Verification items for the finished model (mm, model axes). A direction names the side the tool comes from. Give positions to 0.01 mm unless a question says otherwise; leave off trailing zeros. Loops run counter-clockwise (first coordinate to the right, second up) from the corner with the lowest first, then second, coordinate; pieces in that order, holes last. Notation, with made-up numbers: (89, 30.5) - (134, 30.5) arc R16 ccw to (134, 37.5) - close; hole circle Ø6 at (67, 81). An arc over 180 degrees is marked (long way). One line per question, with ' | ' between items. Start each with the question number.
1. Depth check by flat-ended pin: pin 1 Ø4 at (x, y) = (-2, 11) entering from -Z; pin 2 Ø3.5 at (x, z) = (-10.5, 11) entering from -Y; pin 3 Ø6 at (x, y) = (-8, -2) entering from +Z; pin 4 Ø5.5 at (x, z) = (-11, 11.5) entering from +Y. Enter the tip coordinate at first touch or a pass-through.
2. Thickness scan on line 1 along Y through (x, z) = (-14.5, 1.25); line 2 along Y through (x, z) = (2, 7); line 3 along Y through (x, z) = (-2.5, 6). Record the ranges inside material, lowest first. Write a range as from..to.
3. Section check D-D, the plane y = 0. Enter the section's corners in (x, z), then the cut area to 3 significant figures.
4. Section check C-C, the plane z = 18.25. Enter the section's corners in (x, y), then the cut area to 3 significant figures.
5. Section check A-A, the plane y = 12.5. Enter the section's corners in (x, z) (3 decimals).
6. Mould release check, pull along Y, two halves, no side actions. Record for faces 1 (the face through (-9, 13.5, 10)), 2 (the face through (-17.5, 0, 1)), 3 (the face through (6, -10.25, 13)), 4 (the face through (-14, 14, 1.5)): +Y half, -Y half, draft (parallel to the pull), parting line (faces both ways), or undercut.
7. Section check B-B, the plane x = -10.5. Enter the section's corners in (y, z) (3 decimals), then the cut area to 3 significant figures.
8. Tool access check on faces 5 (the face through (6, 8, 5)), 6 (the face through (-12.517, 12.24, 0.74)), 7 (the face through (-7.7, -14.2, 13.1)). Record the directions out of +Z, -Z, +X, -X, +Y, -Y that give a thin tool (end or side, any length) a straight path to the whole face; none if there is none.
from build123d import *

# Parameters (mm, degrees)
SKETCH1_W              = 35
SKETCH1_H              = 20
BASE_PLATE_DEPTH       = 3
SKETCH2_W              = 35
SKETCH2_H              = 5
SIDE_WALLS_DEPTH       = 23
SKETCH4_R              = 1.1
SKETCH4_R_2            = 1.25
M2_SCREWS_DEPTH        = 23
SKETCH6_W              = 5
SKETCH6_H              = 20
RETURN_STOPPER_DEPTH   = 4.5
SKETCH9_W              = 12
SKETCH9_H              = 16
BOSS_EXTRUDE1_DEPTH    = 4.5
SKETCH7_R              = 7.75
MAGNET_POCKET_DEPTH    = 6
SKETCH8_R              = 2
M2_SCREW_HEAD_DEPTH    = 1.5
M3_ACHSLE_DEPTH        = 39.213217609
M3_ACHSLE_DEPTH_BACK   = 39.213217609
SKETCH5_R              = 1.625
SKETCH14_R             = 3.5
CUT_EXTRUDE1_DEPTH     = 1.5
CUT_EXTRUDE2_START     = -1.5
SKETCH15_R             = 3.5
CUT_EXTRUDE2_DEPTH     = 1.5
FILLET1_R              = 1.5
LEAVER_START           = -0.25
SKETCH11_W             = 22
SKETCH11_H             = 15.5
LEAVER_SPACE_DEPTH     = 20.5
SKETCH12_W             = 17
SKETCH12_H             = 4.5
MORE_SPACE_LEFT_DEPTH  = 0.25
SKETCH13_W             = 17
SKETCH13_H             = 4.5
MORE_SPACE_RIGHT_DEPTH = 0.25
FILLET2_R              = 0.75
FILLET3_R              = 0.75
FILLET4_R              = 0.75
FILLET5_R              = 0.5
CHAMFER1_SIZE          = 13.050517742
CHAMFER1_SIZE_2        = 4.75


with BuildPart() as part:
    # Sketch1 → Base Plate (new body)
    with BuildSketch(Plane.XY):
        Rectangle(SKETCH1_W, SKETCH1_H)
    extrude(amount=BASE_PLATE_DEPTH)

    # Sketch2 → Side Walls (add)
    with BuildSketch(Plane(origin=(0, 0, 0), x_dir=(1, 0, 0), z_dir=(0, 0, -1))):
        with Locations((0, -12.5)):
            Rectangle(SKETCH2_W, SKETCH2_H)
        with Locations((0, 12.5)):
            Rectangle(SKETCH2_W, SKETCH2_H)
    extrude(amount=-SIDE_WALLS_DEPTH)

    # Sketch4 → M2 Screws (cut)
    with BuildSketch(Plane.XY.offset(23)):
        with Locations((-14.5, -12.5)):
            Circle(SKETCH4_R)
        with Locations((7.5, -12.5)):
            Circle(SKETCH4_R)
        with Locations((7.5, 12.5)):
            Circle(SKETCH4_R_2)
        with Locations((-14.5, 12.5)):
            Circle(SKETCH4_R_2)
    extrude(amount=-M2_SCREWS_DEPTH, mode=Mode.SUBTRACT)

    # Sketch6 → Return Stopper (add)
    with BuildSketch(Plane.XY.offset(3)):
        with Locations((15, 0)):
            Rectangle(SKETCH6_W, SKETCH6_H)
    extrude(amount=RETURN_STOPPER_DEPTH)

    # Sketch9 → Boss-Extrude1 (add)
    with BuildSketch(Plane.XY.offset(3)):
        with Locations((6.5, 0)):
            Rectangle(SKETCH9_W, SKETCH9_H)
    extrude(amount=BOSS_EXTRUDE1_DEPTH)

    # Sketch7 → Magnet Pocket (cut)
    with BuildSketch(Plane(origin=(0, 0, 0), x_dir=(-1, 0, 0), z_dir=(0, 0, 1))):
        with Locations(Location((-8.75, 0, 0), (0, 0, 90))):
            Circle(SKETCH7_R)
    extrude(amount=MAGNET_POCKET_DEPTH, mode=Mode.SUBTRACT)

    # Sketch8 → M2 Screw Head (cut)
    with BuildSketch(Plane(origin=(0, 0, 0), x_dir=(1, 0, 0), z_dir=(0, 0, -1))):
        with Locations(Location((7.5, -12.5, 0), (0, 0, 270))):
            Circle(SKETCH8_R)
        with Locations(Location((-14.5, -12.5, 0), (0, 0, 270))):
            Circle(SKETCH8_R)
        with Locations(Location((7.5, 12.5, 0), (0, 0, 270))):
            Circle(SKETCH8_R)
        with Locations(Location((-14.5, 12.5, 0), (0, 0, 270))):
            Circle(SKETCH8_R)
    extrude(amount=-M2_SCREW_HEAD_DEPTH, mode=Mode.SUBTRACT)

    # Sketch5 → M3 Achsle (cut, two sides: drawn at the far end of the back side and taken through both)
    with BuildSketch(Plane.XZ.offset(-10).offset(-M3_ACHSLE_DEPTH_BACK)):
        with Locations((-10.5, 11)):
            Circle(SKETCH5_R)
    extrude(amount=M3_ACHSLE_DEPTH + M3_ACHSLE_DEPTH_BACK, mode=Mode.SUBTRACT)

    # Sketch14 → Cut-Extrude1 (cut)
    with BuildSketch(Plane(origin=(0, 15, 0), x_dir=(-1, 0, 0), z_dir=(0, 1, 0))):
        with Locations((10.5, 11)):
            Circle(SKETCH14_R)
    extrude(amount=-CUT_EXTRUDE1_DEPTH, mode=Mode.SUBTRACT)

    # Sketch15 → Cut-Extrude2 (cut)
    with BuildSketch(Plane.XZ.offset(15).offset(CUT_EXTRUDE2_START)):
        with Locations(Location((-10.5, 11, 0), (0, 0, 180))):
            Circle(SKETCH15_R)
    extrude(amount=CUT_EXTRUDE2_DEPTH, mode=Mode.SUBTRACT)

    # Fillet1
    fillet1_edges = [part.edges().sort_by_distance(p)[0] for p in [
        (0.5, 0, 7.5),
    ]]
    fillet(fillet1_edges, radius=FILLET1_R)

    # Sketch11 → Leaver Space (cut)
    with BuildSketch(Plane.XZ.offset(-10).offset(LEAVER_START)):
        with Locations((6.5, 15.25)):
            Rectangle(SKETCH11_W, SKETCH11_H)
    extrude(amount=LEAVER_SPACE_DEPTH, mode=Mode.SUBTRACT)

    # Sketch12 → More Space left (cut)
    with BuildSketch(Plane.XZ.offset(-10)):
        with Locations((4, 5.25)):
            Rectangle(SKETCH12_W, SKETCH12_H)
    extrude(amount=-MORE_SPACE_LEFT_DEPTH, mode=Mode.SUBTRACT)

    # Sketch13 → More Space right (cut)
    with BuildSketch(Plane(origin=(0, -10, 0), x_dir=(-1, 0, 0), z_dir=(0, 1, 0))):
        with Locations((-4, 5.25)):
            Rectangle(SKETCH13_W, SKETCH13_H)
    extrude(amount=-MORE_SPACE_RIGHT_DEPTH, mode=Mode.SUBTRACT)

    # Fillet2
    # the kernel refuses this fillet: 0.75 mm, written as the material it takes off along each edge
    with BuildSketch(Plane(origin=(19.375, 15, 0), x_dir=(0, -1, 0), z_dir=(-1, 0, 0))) as fillet2_piece_1:
        with BuildLine():
            CenterArc((FILLET2_R, FILLET2_R), FILLET2_R, 180, 90)
            Line((0, FILLET2_R), (0, 0))
            Line((0, 0), (FILLET2_R, 0))
        make_face()
    extrude(amount=38.75, mode=Mode.SUBTRACT)

    # Fillet3
    # the kernel refuses this fillet: 0.75 mm, written as the material it takes off along each edge
    with BuildSketch(Plane(origin=(-19.375, -15, 0), x_dir=(0, 1, 0), z_dir=(1, 0, 0))) as fillet3_piece_1:
        with BuildLine():
            CenterArc((FILLET3_R, FILLET3_R), FILLET3_R, 180, 90)
            Line((0, FILLET3_R), (0, 0))
            Line((0, 0), (FILLET3_R, 0))
        make_face()
    extrude(amount=38.75, mode=Mode.SUBTRACT)

    # Fillet4
    fillet4_edges = [part.edges().sort_by_distance(p)[0] for p in [
        (-17.5, -15, 11.875),
        (-17.5, 0, 0),
        (-17.5, 14.780330086, 0.219669914),
        (-17.5, -14.780330086, 0.219669914),
        (-17.5, 15, 11.875),
    ]]
    fillet(fillet4_edges, radius=FILLET4_R)

    # Fillet5
    fillet5_edges = [part.edges().sort_by_distance(p)[0] for p in [
        (17.5, -15, 11.875),
        (17.5, 14.780330086, 0.219669914),
        (17.5, 0, 0),
        (17.5, -14.780330086, 0.219669914),
        (17.5, 15, 11.875),
    ]]
    fillet(fillet5_edges, radius=FILLET5_R)

    # Chamfer1
    # the kernel refuses this chamfer: 13.050517742, 4.75 mm, written as the material it takes off along each edge
    with BuildSketch(Plane(origin=(17.5, -48.355584384, 23), x_dir=(0.013184058198645798, 0, -0.9999130865277316), z_dir=(0, 1, 0))) as chamfer1_piece_1:
        Polygon((CHAMFER1_SIZE * 0.999913086559, CHAMFER1_SIZE * 0.0131840581991), (-CHAMFER1_SIZE_2 * 0.0131840581986, CHAMFER1_SIZE_2 * 0.999913086528), (0, 0), align=None)
    extrude(amount=71.961168769, mode=Mode.SUBTRACT)
    with BuildSketch(Plane(origin=(17.5, -23.605584384, 23), x_dir=(-0.9950833631817486, 0, 0.09904090225205059), z_dir=(0, 1, 0))) as chamfer1_piece_2:
        Polygon((CHAMFER1_SIZE_2 * 0.995083363182, -CHAMFER1_SIZE_2 * 0.0990409022521), (-CHAMFER1_SIZE * 0.0990409022552, -CHAMFER1_SIZE * 0.995083363213), (0, 0), align=None)
    extrude(amount=71.961168769, mode=Mode.SUBTRACT)


solid = part.part
Results list:
1) pin 1: z = 0 | pin 2: y = -13.5 | pin 3: z = 3 | pin 4: y = 13.5
2) line 1: -15..-14.5, -10.5..10.5, 14.5..15 | line 2: -15..-10.25, -8..8, 10.25..15 | line 3: -15..-10.25, 10.25..15
3) outline: (-17.5, 0.75) arc R0.75 ccw to (-16.75, 0) - (1, 0) - (1, 6) - (16.5, 6) - (16.5, 0) - (17, 0) arc R0.5 ccw to (17.5, 0.5) - (17.5, 7.5) - (2, 7.5) arc R1.5 ccw to (0.5, 6) - (0.5, 3) - (-17.5, 3) - close | area: 87.8 mm²
4) outline: (-17.5, -14.25) arc R0.75 ccw to (-16.75, -15) - (14.48, -15) - (14.48, -10.25) - (-4.5, -10.25) - (-4.5, -10) - (-17.5, -10) - close; (-17.5, 10) - (-4.5, 10) - (-4.5, 10.25) - (14.48, 10.25) - (14.48, 15) - (-16.75, 15) arc R0.75 ccw to (-17.5, 14.25) - close; hole circle Ø2.5 at (-14.5, 12.5); hole circle Ø2.2 at (-14.5, -12.5); hole circle Ø2.5 at (7.5, 12.5); hole circle Ø2.2 at (7.5, -12.5) | area: 293 mm²
5) outline: (-17.5, 0.75) arc R0.75 ccw to (-16.75, 0) - (-16.5, 0) - (-16.5, 1.5) - (-15.75, 1.5) - (-15.75, 23) - (-17.5, 23) - close; (-13.25, 1.5) - (-12.5, 1.5) - (-12.5, 0) - (5.5, 0) - (5.5, 1.5) - (6.25, 1.5) - (6.25, 23) - (-13.25, 23) - close; (8.75, 1.5) - (9.5, 1.5) - (9.5, 0) - (17, 0) arc R0.5 ccw to (17.5, 0.5) - (17.5, 9.949) - (12.75, 23) - (8.75, 23) - close; hole circle Ø3.25 at (-10.5, 11)
6) face 1: +Y half | face 2: draft | face 3: undercut | face 4: undercut
7) outline: (-15, 0.75) arc R0.75 ccw to (-14.25, 0) - (14.25, 0) arc R0.75 ccw to (15, 0.75) - (15, 7.5) - (13.5, 7.5) - (13.5, 9.375) - (10, 9.375) - (10, 3) - (-10, 3) - (-10, 9.375) - (-13.5, 9.375) - (-13.5, 7.5) - (-15, 7.5) - close; (-15, 14.5) - (-13.5, 14.5) - (-13.5, 12.625) - (-10, 12.625) - (-10, 23) - (-15, 23) - close; (10, 12.625) - (13.5, 12.625) - (13.5, 14.5) - (15, 14.5) - (15, 23) - (10, 23) - close | area: 246 mm²
8) face 5: +Z, -X | face 6: -Z | face 7: -Y
